from build123d import *

# Parameters (mm, degrees)
F0_R     = 16
F0_R_2   = 6
F1_DEPTH = 15.9
F2_R     = 0.6
F3_R     = 13.85
F3_R_2   = 8.6
F4_DEPTH = 0.5
F5_R     = 13.85
F5_R_2   = 8.6
F6_DEPTH = 0.5


with BuildPart() as f1:
    # F0 (on Top) → F1 (new body)
    with BuildSketch(Plane.XY):
        Circle(F0_R)
        Circle(F0_R_2, mode=Mode.SUBTRACT)
    extrude(amount=F1_DEPTH)

    # F2
    f2_edges = [f1.edges().sort_by_distance(p)[0] for p in [
        (6, 0, 7.95),
        (-6, 0, 0),
        (-6, 0, 15.9),
        (16, 0, 7.95),
        (-16, 0, 0),
        (-16, 0, 15.9),
    ]]
    fillet(f2_edges, radius=F2_R)

    # F3 (on face) → F4 (cut)
    with BuildSketch(Plane.XY.offset(15.9)):
        Circle(F3_R)
        Circle(F3_R_2, mode=Mode.SUBTRACT)
    extrude(amount=-F4_DEPTH, mode=Mode.SUBTRACT)

    # F5 (on face) → F6 (cut)
    with BuildSketch(Plane(origin=(0, 0, 0), x_dir=(1, 0, 0), z_dir=(0, 0, -1))):
        Circle(F5_R)
        Circle(F5_R_2, mode=Mode.SUBTRACT)
    extrude(amount=-F6_DEPTH, mode=Mode.SUBTRACT)


solid = f1.part
Read the model definition and answer for the solid it produces. Units are mm, in the model's axes. A direction names the side the tool comes from. Round coordinates to 2 decimals unless told otherwise and drop trailing zeros. Order: outer loops, then holes, each group sorted by start corner. A loop starts at its lowest first (then second) coordinate and runs counter-clockwise, first axis right, second up. Notation, with made-up numbers: (73, 60.5) - (121, 60.5) arc R32 ccw to (121, 95.5) - close; hole circle Ø3 at (37.5, 71.25). An arc over 180 degrees is marked (long way). Use one line per item in the form item = value. Start each with the question number.
(1) The part is cut by section C-C (z = 11). Give the vertices of the cut face in (x, y).
(2) For faces 1 (the face through (13.21, 4.16, 15.65)), 2 (the face through (-13, 6, 15.9)), 3 (the face through (-8.59, -0.38, 0.25)), determine the directions among +Z, -Z, +X, -X, +Y, -Y from which every point of the face is accessible in a straight line to the end or side of a thin tool.
(3) Flat-ended cylindrical pins translate along their axes: pin 1 Ø5 at (x, z) = (-5, 13.5) entering from -Y; pin 2 Ø3 at (y, z) = (-8, 13.5) entering from -X; pin 3 Ø3 at (y, z) = (-1, 12.5) entering from +X; pin 4 Ø2 at (x, y) = (-10, -6) entering from -Z. Find the tip coordinate at first contact, or state that the pin passes through.
(4) Find the intervals of material crossed by line 1 along Y through (x, z) = (0, 11); line 2 along Y through (x, z) = (0, 15.7); line 3 along Y through (x, z) = (0, 0.45), in increasing order. Write a range as from..to.
Checked values:
q1.outline = circle Ø32 at (0, 0); hole circle Ø12 at (0, 0)
q2.face_1 = +Z
q2.face_2 = +Z, +X, -X, +Y, -Y
q2.face_3 = -Z
q3.pin_1 = -15.8
q3.pin_2 = -14.62
q3.pin_3 = 16
q3.pin_4 = 0.5
q4.line_1 = -16..-6, 6..16
q4.line_2 = -15.85..-13.85, -8.6..-6.15, 6.15..8.6, 13.85..15.85
q4.line_3 = -15.98..-13.85, -8.6..-6.02, 6.02..8.6, 13.85..15.98
